For this review, take the finished solid that the model builds, in its own axes (mm). A direction names the side the tool comes from. Round coordinates to 2 decimals unless told otherwise and drop trailing zeros. Write each loop counter-clockwise with the first axis right and the second up, starting at its lowest first coordinate (ties: lowest second). Pieces come first, ordered by that corner, then holes.
from build123d import *

# Parameters (mm, degrees)
SKETCH1_R           = 60
SKETCH1_R_2         = 2.65
BOSS_EXTRUDE2_DEPTH = 2
CUT_EXTRUDE1_DEPTH  = 85.876380696
CIRPATTERN1_COUNT   = 6
SKETCH3_R           = 4.65
SKETCH3_R_2         = 2.65
BOSS_EXTRUDE3_DEPTH = 5.5
CHAMFER1_SIZE       = 2
CHAMFER1_SIZE2      = 5


with BuildPart() as part:
    # Sketch1 → Boss-Extrude2 (new body)
    with BuildSketch(Plane.XY):
        Circle(SKETCH1_R)
        with BuildLine():
            ThreePointArc((40, -30), (0, -50), (-40, -30))
            ThreePointArc((-40, -30), (0, -10), (40, -30))
        make_face(mode=Mode.SUBTRACT)
        with BuildLine():
            ThreePointArc((-5.980762114, 49.641016151), (-8.660254038, 5), (-45.980762114, -19.641016151))
            ThreePointArc((-45.980762114, -19.641016151), (-43.301270189, 25), (-5.980762114, 49.641016151))
        make_face(mode=Mode.SUBTRACT)
        Circle(SKETCH1_R_2, mode=Mode.SUBTRACT)
        with BuildLine():
            ThreePointArc((5.980762114, 49.641016151), (43.301270189, 25), (45.980762114, -19.641016151))
            ThreePointArc((45.980762114, -19.641016151), (8.660254038, 5), (5.980762114, 49.641016151))
        make_face(mode=Mode.SUBTRACT)
    extrude(amount=BOSS_EXTRUDE2_DEPTH)

    # Sketch2 → Cut-Extrude1 (cut, through all)
    with BuildSketch(Plane.XY.offset(2)):
        with BuildLine():
            ThreePointArc((0, 57.1), (-2.1, 55), (0, 52.9))
            Line((0, 52.9), (0, 57.1))
        make_face()
        with BuildLine():
            Line((0, 57.1), (0, 52.9))
            ThreePointArc((0, 52.9), (1.48492424, 53.51507576), (2.1, 55))
            ThreePointArc((2.1, 55), (1.48492424, 56.48492424), (0, 57.1))
        make_face()
    cut_extrude1 = extrude(amount=-CUT_EXTRUDE1_DEPTH, mode=Mode.SUBTRACT)

    # CirPattern1: Cut-Extrude1 ×6 about axis
    cirpattern1_axis = Axis((0, 0, 0), (0, 0, 1))
    for i in range(1, CIRPATTERN1_COUNT):
        add(cut_extrude1.rotate(cirpattern1_axis, i * 360 / CIRPATTERN1_COUNT), mode=Mode.SUBTRACT)

    # Sketch3 → Boss-Extrude3 (add)
    with BuildSketch(Plane.XY.offset(2)):
        Circle(SKETCH3_R)
        Circle(SKETCH3_R_2, mode=Mode.SUBTRACT)
    extrude(amount=BOSS_EXTRUDE3_DEPTH)

    # Chamfer1
    chamfer1_edges = [part.edges().sort_by_distance(p)[0] for p in [
        (-4.65, 0, 2),
    ]]
    chamfer1_side = [part.faces().sort_by_distance(p)[0] for p in [
        (-58.302943725, 0, 2),
    ]]
    chamfer(chamfer1_edges, length=CHAMFER1_SIZE, length2=CHAMFER1_SIZE2, reference=chamfer1_side[0])


solid = part.part
(1) We need section C-C, the plane z = 4.75. Give the boundary of the cut face in (x, y), and give its area (3 significant figures).
Geometry check:
outline: circle Ø11.1 at (0, 0); hole circle Ø5.3 at (0, 0)
area: 74.7 mm2
(2) For line 1 along Y through (x, z) = (0, 3.75); line 2 along Z through (x, y) = (38, 36.5); line 3 along Y through (x, z) = (0, 4.25), list the stretches that pass through material, from the lowest coordinate up.
Geometry check:
line 1: y = -5.95 to -2.65, 2.65 to 5.95
line 2: z = 0 to 2
line 3: y = -5.75 to -2.65, 2.65 to 5.75
(3) We need section D-D, the plane y = -37.5. Give the boundary of the cut face in (x, z), and give its area (3 significant figures).
Geometry check:
outline: (-46.84, 0) - (-33.07, 0) - (-33.07, 2) - (-46.84, 2) - close; (33.07, 0) - (46.84, 0) - (46.84, 2) - (33.07, 2) - close
area: 55.1 mm2
(4) We need section B-B, the plane y = 41.5. Give the boundary of the cut face in (x, z).
Geometry check:
outline: (-43.33, 0) - (-27.89, 0) - (-27.89, 2) - (-43.33, 2) - close; (-3.3, 0) - (3.3, 0) - (3.3, 2) - (-3.3, 2) - close; (27.89, 0) - (43.33, 0) - (43.33, 2) - (27.89, 2) - close
(5) For pin 1 Ø8.5 at (x, y) = (0, 0) entering from +Z; pin 2 Ø1 at (y, z) = (-46.5, 2) entering from -X, all flat-tipped, find the tip position at first contact; note any pin that passes through.
Geometry check:
pin 1: stops at z = 7.5
pin 2: stops at x = -38.52
(6) We need section A-A, the plane x = 20. Give the boundary of the cut face in (y, z), and give its area (3 significant figures).
Geometry check:
outline: (-56.57, 0) - (-45.83, 0) - (-45.83, 2) - (-56.57, 2) - close; (-14.17, 0) - (-8.45, 0) - (-8.45, 2) - (-14.17, 2) - close; (45.83, 0) - (56.57, 0) - (56.57, 2) - (45.83, 2) - close
area: 54.4 mm2
(7) For faces 1 (the face through (4.74, 1.49, 6.2)), 2 (the face through (-8.34, 5.56, 0.99)), list the 3-axis set-ups (+Z, -Z, +X, -X, +Y, -Y) from which the entire face can be reached by the end or side of a thin tool; tool diameter is ignored.
Geometry check:
face 1: +Z
face 2: +Z, -Z
(8) Mouldability with a two-part tool opening along Y and no side actions: class faces 3 (the face through (2.5, 3.92, 7.25)), 4 (the face through (8.99, 4.44, 0.99)), 5 (the face through (-5, 0, 0)) as pulls with the +Y half, pulls with the -Y half, needs draft (parallel to the pull), parting line crosses it, or undercut.
Geometry check:
face 3: parting line crosses it
face 4: undercut
face 5: needs draft
